from build123d import *

# Parameters (mm, degrees)
SKETCH_1_W          = 20
SKETCH_1_H          = 20
SKETCH_1_W_2        = 18
SKETCH_1_H_2        = 18
EXTRUDE_1_DEPTH     = 200
SKETCH_3_R          = 1.6
CUT_EXTRUDE_1_DEPTH = 202.246117975
CUT_EXTRUDE_2_REACH = 203.246


with BuildPart() as part:
    # 草图1 → 凸台-拉伸1 (new body)
    with BuildSketch(Plane.XY):
        Rectangle(SKETCH_1_W, SKETCH_1_H)
        Rectangle(SKETCH_1_W_2, SKETCH_1_H_2, mode=Mode.SUBTRACT)
    extrude(amount=EXTRUDE_1_DEPTH)

    # 草图3 → 切除-拉伸1 (cut, through all)
    with BuildSketch(Plane(origin=(0, 10, 0), x_dir=(1, 0, 0), z_dir=(0, 1, 0))):
        with Locations(Location((-4.5, -134.5, 0), (0, 0, 270))):
            Circle(SKETCH_3_R)
        with Locations(Location((4.5, -134.5, 0), (0, 0, 270))):
            Circle(SKETCH_3_R)
        with Locations(Location((4.5, -125.5, 0), (0, 0, 270))):
            Circle(SKETCH_3_R)
        with Locations(Location((-4.5, -125.5, 0), (0, 0, 270))):
            Circle(SKETCH_3_R)
        with Locations(Location((4.5, -65.5, 0), (0, 0, 270))):
            Circle(SKETCH_3_R)
        with Locations(Location((4.5, -74.5, 0), (0, 0, 270))):
            Circle(SKETCH_3_R)
        with Locations(Location((-4.5, -74.5, 0), (0, 0, 270))):
            Circle(SKETCH_3_R)
        with Locations(Location((-4.5, -65.5, 0), (0, 0, 270))):
            Circle(SKETCH_3_R)
        with Locations(Location((-4.5, -184.5, 0), (0, 0, 270))):
            Circle(SKETCH_3_R)
        with Locations(Location((4.5, -184.5, 0), (0, 0, 270))):
            Circle(SKETCH_3_R)
        with Locations(Location((4.5, -175.5, 0), (0, 0, 270))):
            Circle(SKETCH_3_R)
        with Locations(Location((-4.5, -175.5, 0), (0, 0, 270))):
            Circle(SKETCH_3_R)
        with Locations(Location((-4.5, -24.5, 0), (0, 0, 270))):
            Circle(SKETCH_3_R)
        with Locations(Location((4.5, -24.5, 0), (0, 0, 270))):
            Circle(SKETCH_3_R)
        with Locations(Location((4.5, -15.5, 0), (0, 0, 270))):
            Circle(SKETCH_3_R)
        with Locations(Location((-4.5, -15.5, 0), (0, 0, 270))):
            Circle(SKETCH_3_R)
    extrude(amount=-CUT_EXTRUDE_1_DEPTH, mode=Mode.SUBTRACT)

    # 草图4 → 切除-拉伸2 (cut, up to next)
    with BuildSketch(Plane(origin=(0, 10, 0), x_dir=(1, 0, 0), z_dir=(0, 1, 0)), mode=Mode.PRIVATE) as cut_extrude_2_sk1:
        with BuildLine():
            Line((4.5, -11), (-4.5, -11))
            ThreePointArc((-4.5, -11), (-7.681980515, -12.318019485), (-9, -15.5))
            Line((-9, -15.5), (-9, -24.5))
            ThreePointArc((-9, -24.5), (-7.681980515, -27.681980515), (-4.5, -29))
            Line((-4.5, -29), (4.5, -29))
            ThreePointArc((4.5, -29), (7.681980515, -27.681980515), (9, -24.5))
            Line((9, -24.5), (9, -15.5))
            ThreePointArc((9, -15.5), (7.681980515, -12.318019485), (4.5, -11))
        make_face()
    cut_extrude_2_tool1 = extrude(cut_extrude_2_sk1.sketch, amount=-CUT_EXTRUDE_2_REACH, mode=Mode.PRIVATE) & part.part
    # 草图4 → 切除-拉伸2 (cut, up to next)
    with BuildSketch(Plane(origin=(0, 10, 0), x_dir=(1, 0, 0), z_dir=(0, 1, 0)), mode=Mode.PRIVATE) as cut_extrude_2_sk2:
        with BuildLine():
            Line((4.5, -79), (-4.5, -79))
            ThreePointArc((-4.5, -79), (-7.681980515, -77.681980515), (-9, -74.5))
            Line((-9, -74.5), (-9, -65.5))
            ThreePointArc((-9, -65.5), (-7.681980515, -62.318019485), (-4.5, -61))
            Line((-4.5, -61), (4.5, -61))
            ThreePointArc((4.5, -61), (7.681980515, -62.318019485), (9, -65.5))
            Line((9, -65.5), (9, -74.5))
            ThreePointArc((9, -74.5), (7.681980515, -77.681980515), (4.5, -79))
        make_face()
    cut_extrude_2_tool2 = extrude(cut_extrude_2_sk2.sketch, amount=-CUT_EXTRUDE_2_REACH, mode=Mode.PRIVATE) & part.part
    # 草图4 → 切除-拉伸2 (cut, up to next)
    with BuildSketch(Plane(origin=(0, 10, 0), x_dir=(1, 0, 0), z_dir=(0, 1, 0)), mode=Mode.PRIVATE) as cut_extrude_2_sk3:
        with BuildLine():
            Line((9, -134.5), (9, -125.5))
            ThreePointArc((9, -125.5), (7.681980515, -122.318019485), (4.5, -121))
            Line((4.5, -121), (-4.5, -121))
            ThreePointArc((-4.5, -121), (-7.681980515, -122.318019485), (-9, -125.5))
            Line((-9, -125.5), (-9, -134.5))
            ThreePointArc((-9, -134.5), (-7.681980515, -137.681980515), (-4.5, -139))
            Line((-4.5, -139), (4.5, -139))
            ThreePointArc((4.5, -139), (7.681980515, -137.681980515), (9, -134.5))
        make_face()
    cut_extrude_2_tool3 = extrude(cut_extrude_2_sk3.sketch, amount=-CUT_EXTRUDE_2_REACH, mode=Mode.PRIVATE) & part.part
    # 草图4 → 切除-拉伸2 (cut, up to next)
    with BuildSketch(Plane(origin=(0, 10, 0), x_dir=(1, 0, 0), z_dir=(0, 1, 0)), mode=Mode.PRIVATE) as cut_extrude_2_sk4:
        with BuildLine():
            Line((9, -184.5), (9, -175.5))
            ThreePointArc((9, -175.5), (7.681980515, -172.318019485), (4.5, -171))
            Line((4.5, -171), (-4.5, -171))
            ThreePointArc((-4.5, -171), (-7.681980515, -172.318019485), (-9, -175.5))
            Line((-9, -175.5), (-9, -184.5))
            ThreePointArc((-9, -184.5), (-7.681980515, -187.681980515), (-4.5, -189))
            Line((-4.5, -189), (4.5, -189))
            ThreePointArc((4.5, -189), (7.681980515, -187.681980515), (9, -184.5))
        make_face()
    cut_extrude_2_tool4 = extrude(cut_extrude_2_sk4.sketch, amount=-CUT_EXTRUDE_2_REACH, mode=Mode.PRIVATE) & part.part
    add(cut_extrude_2_tool1.solids().sort_by_distance((0, 10, 20))[0], mode=Mode.SUBTRACT)
    add(cut_extrude_2_tool2.solids().sort_by_distance((0, 10, 70))[0], mode=Mode.SUBTRACT)
    add(cut_extrude_2_tool3.solids().sort_by_distance((0, 10, 130))[0], mode=Mode.SUBTRACT)
    add(cut_extrude_2_tool4.solids().sort_by_distance((0, 10, 180))[0], mode=Mode.SUBTRACT)


solid = part.part
Could you check a few things on this model? Use its own coordinates, in mm. A direction names the side the tool comes from. Give positions to 0.01 mm unless a question says otherwise; leave off trailing zeros. Order: outer loops, then holes, each group sorted by start corner. A loop starts at its lowest first (then second) coordinate and runs counter-clockwise, first axis right, second up. Notation, with made-up numbers: (-16.5, -28) -> (37.5, -28) arc R5 ccw to (37.5, -19) -> close; hole circle Ø11 at (40.25, -22). An arc over 180 degrees is marked (long way). Answer in a Markdown table with one row per item. Add a question column.
Item 1: We'd pull the mould along Y, two halves only. Please class faces 4 (the cylindrical face through (7.717, 9.507, 77.647)), 5 (the flat face through (0, -9, 99)), 6 (the flat face through (0, -10, 99)): pulls with the +Y half, pulls with the -Y half, needs draft (parallel to the pull), parting line crosses it, or undercut.
Item 2: Imagine slicing it at C-C (z = 40.5). List the corners of the cut face in (x, y) for me.
Item 3: Please list where these lines run through material, in increasing order: probe 1 along X at (y, z) = (-9.35, 125.5); probe 2 along X at (y, z) = (-8, 100).
Item 4: For faces 1 (the flat face through (0, 9, 100)), 2 (the cylindrical face through (-7.647, 9.507, 122.283)), 3 (the cylindrical face through (-4.019, -9.493, 76.026)), which set-ups out of +Z, -Z, +X, -X, +Y, -Y let a thin tool reach every point of the face, with its end or its side?
Item 5: Imagine slicing it at A-A (y = 7). List the corners of the cut face in (x, z) for me, and give its area (3 significant figures).
Item 6: I'm going to push flat-ended pins straight in: P1, Ø1.9, axis at x = 4.5, z = 15.5, coming from the +Y side; P2, Ø4, axis at x = -1.5, z = 25, coming from the +Y side. Where does each tip first touch, or does it pass through?
Item 7: Imagine slicing it at B-B (x = 0.5). List the corners of the cut face in (y, z) for me.
Result:
| question | item | result |
|---|---|---|
| 1 | face 4 | needs draft |
| 1 | face 5 | undercut |
| 1 | face 6 | pulls with the -Y half |
| 2 | outline | (-10, -10) -> (10, -10) -> (10, 10) -> (-10, 10) -> close; hole (-9, -9) -> (9, -9) -> (9, 9) -> (-9, 9) -> close |
| 3 | probe 1 | -10 to -6.1, -2.9 to 2.9, 6.1 to 10 |
| 3 | probe 2 | -10 to -9, 9 to 10 |
| 4 | face 1 | +Z, -Z |
| 4 | face 2 | +Y |
| 4 | face 3 | +Y, -Y |
| 5 | outline | (-10, 0) -> (-9, 0) -> (-9, 200) -> (-10, 200) -> close; (9, 0) -> (10, 0) -> (10, 200) -> (9, 200) -> close |
| 5 | area | 400 mm2 |
| 6 | P1 | through |
| 6 | P2 | y = -9 |
| 7 | outline | (-10, 0) -> (-9, 0) -> (-9, 200) -> (-10, 200) -> close; (9, 0) -> (10, 0) -> (10, 11) -> (9, 11) -> close; (9, 29) -> (10, 29) -> (10, 61) -> (9, 61) -> close; (9, 79) -> (10, 79) -> (10, 121) -> (9, 121) -> close; (9, 139) -> (10, 139) -> (10, 171) -> (9, 171) -> close; (9, 189) -> (10, 189) -> (10, 200) -> (9, 200) -> close |
